```python
from build123d import *

# Parameters (mm, degrees)
SKETCH_1_R      = 1.6
EXTRUDE_1_DEPTH = 3
FILLET_1_R      = 5
EXTRUDE_2_DEPTH = 3
FILLET_2_R      = 3


with BuildPart() as part:
    # 草图1 → 凸台-拉伸1 (new body)
    with BuildSketch(Plane.XY):
        Polygon((-40, 0), (-40, 20), (40, 20), (40, 0), (10, 0), (10, -30), (-10, -30), (-10, 0), align=None)
        with Locations((-30, 10)):
            Circle(SKETCH_1_R, mode=Mode.SUBTRACT)
        with Locations((-20, 10)):
            Circle(SKETCH_1_R, mode=Mode.SUBTRACT)
        with Locations((0, -10)):
            Circle(SKETCH_1_R, mode=Mode.SUBTRACT)
        with Locations((0, -20)):
            Circle(SKETCH_1_R, mode=Mode.SUBTRACT)
        with Locations((20, 10)):
            Circle(SKETCH_1_R, mode=Mode.SUBTRACT)
        with Locations((30, 10)):
            Circle(SKETCH_1_R, mode=Mode.SUBTRACT)
    extrude(amount=EXTRUDE_1_DEPTH)

    # 圆角1
    fillet_1_edges = [part.edges().sort_by_distance(p)[0] for p in [
        (-40, 0, 1.5),
        (-40, 20, 1.5),
        (40, 20, 1.5),
        (40, 0, 1.5),
        (10, 0, 1.5),
        (10, -30, 1.5),
        (-10, -30, 1.5),
        (-10, 0, 1.5),
    ]]
    fillet(fillet_1_edges, radius=FILLET_1_R)

    # 草图2 → 凸台-拉伸2 (add)
    with BuildSketch(Plane(origin=(0, 0, 0), x_dir=(-1, 0, 0), z_dir=(0, 0, -1))):
        Polygon((-33.656854249, 0), (-10, -23.656854249), (-10, -18), (-28, 0), align=None)
        Polygon((10, -18), (28, 0), (33.656854249, 0), (10, -23.656854249), align=None)
    extrude(amount=-EXTRUDE_2_DEPTH)

    # 圆角2
    fillet_2_edges = [part.edges().sort_by_distance(p)[0] for p in [
        (33.656854249, 0, 1.5),
        (28, 0, 1.5),
        (10, -18, 1.5),
        (10, -23.656854249, 1.5),
        (-10, -23.656854249, 1.5),
        (-10, -18, 1.5),
        (-28, 0, 1.5),
        (-33.656854249, 0, 1.5),
    ]]
    fillet(fillet_2_edges, radius=FILLET_2_R)


solid = part.part
```
Can you work these out from the model? Positions are in its coordinate system, mm. A direction names the side the tool comes from. Give positions to 0.01 mm unless a question says otherwise; leave off trailing zeros. Loops run counter-clockwise (first coordinate to the right, second up) from the corner with the lowest first, then second, coordinate; pieces in that order, holes last. Notation, with made-up numbers: M 54,54.25 L 82,54.25 A36 ccw 82,92.25 Z; hole C 55.25,25 d9. An arc over 180 degrees is marked long. One line per item, written item: value.
(1) Suppose I cut it at A-A on y = 10. List the corners of the cut face in (x, z) for me.
Returned:
outline: M -40,0 L -31.6,0 L -31.6,3 L -40,3 Z; M -28.4,0 L -21.6,0 L -21.6,3 L -28.4,3 Z; M -18.4,0 L 18.4,0 L 18.4,3 L -18.4,3 Z; M 21.6,0 L 28.4,0 L 28.4,3 L 21.6,3 Z; M 31.6,0 L 40,0 L 40,3 L 31.6,3 Z
(2) I need wall thicknesses on line 1 (Y direction, x = 0, z = 1.6); line 2 (X direction, y = -4, z = 0.45); line 3 (Y direction, x = 19.5, z = 1.65). Which ranges of each line are inside material? Lowest first, please.
Returned:
line 1: -30 to -21.6, -18.4 to -11.6, -8.4 to 20
line 2: -29.66 to -23.59, -10.1 to 10.1, 23.59 to 29.66
line 3: -14.16 to -8.5, 0 to 8.48, 11.52 to 20
(3) Suppose I cut it at C-C on x = 20. List the corners of the cut face in (y, z) for me, plus the area to 3 significant figures.
Returned:
outline: M -13.66,0 L -8,0 L -8,3 L -13.66,3 Z; M 0,0 L 8.4,0 L 8.4,3 L 0,3 Z; M 11.6,0 L 20,0 L 20,3 L 11.6,3 Z
area: 67.4 mm^2
(4) We'd pull the mould along Y, two halves only. Please class faces 3 (the face through (-12, -1, 2)), 4 (the face through (-40, 10, 1)), 5 (the face through (33.77, -0.22, 1.52)): released by +Y, released by -Y, zero draft, split by the parting line, or undercut.
Returned:
face 3: undercut
face 4: zero draft
face 5: released by -Y
(5) Will these pins go through, and if not, where does the flat tip stop? pin 1 (0.9 mm diameter, centred on y = -9, z = 1, fed in from +X); pin 2 (2.5 mm diameter, centred on x = 20, y = 10, fed in from +Z); pin 3 (1.5 mm diameter, centred on x = 17, z = 1.5, fed in from -Y).
Returned:
pin 1: x = 25.11
pin 2: through
pin 3: y = -17.41
(6) Which directions (+Z, -Z, +X, -X, +Y, -Y) give clear straight access to the entire face, cutting with the end or side of a thin tool? Please do faces 1 (the face through (38, 19, 2)), 2 (the face through (12, -1, 2)).
Returned:
face 1: +Z, -Z, +X, +Y
face 2: +Z, -Z
(7) Suppose I cut it at D-D on y = -10. List the corners of the cut face in (x, z) for me, plus the area to 3 significant figures.
Returned:
outline: M -23.66,0 L -18,0 L -18,3 L -23.66,3 Z; M -10,0 L -1.6,0 L -1.6,3 L -10,3 Z; M 1.6,0 L 10,0 L 10,3 L 1.6,3 Z; M 18,0 L 23.66,0 L 23.66,3 L 18,3 Z
area: 84.3 mm^2
(8) Suppose I cut it at B-B on x = -30. List the corners of the cut face in (y, z) for me.
Returned:
outline: M -3.66,0 L 8.4,0 L 8.4,3 L -3.66,3 Z; M 11.6,0 L 20,0 L 20,3 L 11.6,3 Z
